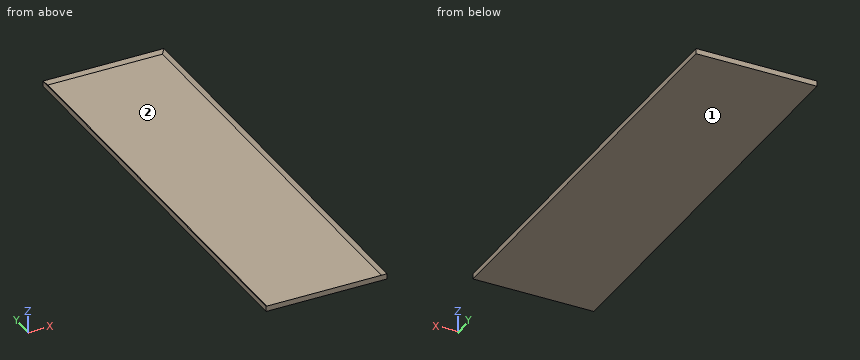
from build123d import *

# Parameters (mm, degrees)
SKETCH2_W           = 560
SKETCH2_H           = 2000
BOSS_EXTRUDE1_DEPTH = 25
SKETCH4_W           = 560
SKETCH4_H           = 2000
CUT_EXTRUDE1_DEPTH  = 15
CUT_EXTRUDE1_DRAFT  = -45


with BuildPart() as part:
    # Sketch2 → Boss-Extrude1 (new body)
    with BuildSketch(Plane.XY):
        with Locations((280, 1000)):
            Rectangle(SKETCH2_W, SKETCH2_H)
    extrude(amount=BOSS_EXTRUDE1_DEPTH)


with BuildPart() as cut_extrude1_tool:
    # Sketch4 → Cut-Extrude1 (with draft: the straight prism first)
    with BuildSketch(Plane.XY.offset(25)):
        with Locations((280, 1000)):
            Rectangle(SKETCH4_W, SKETCH4_H)
    extrude(amount=-CUT_EXTRUDE1_DEPTH)
    # Cut-Extrude1: the draft: its side faces are tilted about the plane it starts from
    cut_extrude1_sides = [cut_extrude1_tool.faces().sort_by_distance(p)[0] for p in [
        (0, 1000, 17.5),
        (280, 0, 17.5),
        (560, 1000, 17.5),
        (280, 2000, 17.5),
    ]]
    draft(cut_extrude1_sides, Plane.XY.offset(25), CUT_EXTRUDE1_DRAFT)


with BuildPart() as part_1:
    add(part.part)

    # Cut-Extrude1: cut by cut_extrude1_tool
    add(cut_extrude1_tool.part, mode=Mode.SUBTRACT)


solid = part_1.part
Verification items for the finished model (mm, model axes). Face numbers are marked on the shaded views. Give positions to 0.01 mm unless a question says otherwise; leave off trailing zeros. Write each loop counter-clockwise with the first axis right and the second up, starting at its lowest first coordinate (ties: lowest second). Pieces come first, ordered by that corner, then holes. Notation, with made-up numbers: (52.5, 42) -> (97.5, 42) arc R14 ccw to (97.5, 47) -> close; hole circle Ø9 at (87, 80.5). An arc over 180 degrees is marked (long way). Use CSV: the item, a comma, the result in double quotes.
(1) Sectioned sample at A-A (z = 20). Record the cut outline in (x, y), plus the area to 3 significant figures.
Derived:
outline,"(0, 0) -> (560, 0) -> (560, 2000) -> (0, 2000) -> close; hole (5, 5) -> (555, 5) -> (555, 1995) -> (5, 1995) -> close"
area,"25,500 mm^2"
(2) Material ranges on L1, parallel to Z at x = 505.5, y = 1861; L2, parallel to Y at x = 513, z = 21.75; L3, parallel to X at y = 649.5, z = 24.25, recorded low to high.
Derived:
L1,"z = 0 to 10"
L2,"y = 0 to 3.25, 1996.75 to 2000"
L3,"x = 0 to 0.75, 559.25 to 560"
(3) Sectioned sample at B-B (y = 1521). Record the cut outline in (x, z), plus the area to 4 significant figures.
Derived:
outline,"(0, 0) -> (560, 0) -> (560, 25) -> (545, 10) -> (15, 10) -> (0, 25) -> close"
area,"5,825 mm^2"
(4) Release check for a two-part mould opening along X. For the marked faces 1 and 2 record: +X half, -X half, draft (parallel to the pull), parting line (faces both ways), or undercut.
Derived:
face 1,"draft"
face 2,"undercut"
(5) Sectioned sample at C-C (x = 376.5). Record the cut outline in (y, z), plus the area to 3 significant figures.
Derived:
outline,"(0, 0) -> (2000, 0) -> (2000, 25) -> (1985, 10) -> (15, 10) -> (0, 25) -> close"
area,"20,200 mm^2"
